Study the drawing (mm; zero at the part's minimum x, y, z) and answer. Round coordinates to 2 decimals unless told otherwise and drop trailing zeros. Write each loop counter-clockwise with the first axis right and the second up, starting at its lowest first coordinate (ties: lowest second). Pieces come first, ordered by that corner, then holes. Notation, with made-up numbers: (87, 0.5) - (96, 0.5) arc R27 ccw to (96, 39.5) - close; hole circle Ø7 at (-16, -8.75). An arc over 180 degrees is marked (long way). Use one line per item in the form item = value. Start each with the question number.
1) The part is cut by section C-C, the plane y = 0.25. Give the vertices of the cut face in (x, z), plus the area to 3 significant figures.
2) This flat-tipped pin is pushed along its axis until it touches: pin 1 (4 mm diameter, centred on x = 30, z = 38.5, fed in from -Y). Where does it stop, or does it pass through?
3) Consider line 1 along Z through (x, y) = (4.5, 0.8); line 2 along Z through (x, y) = (19, 0.95). Determine where each line is inside the solid, lowest interval first. Write a range as from..to.
4) The part is cut by section A-A, the plane x = 4.5. Give the vertices of the cut face in (y, z), plus the area to 3 significant figures.
5) The part is cut by section B-B, the plane z = 3. Give the vertices of the cut face in (x, y).
6) The part is cut by section D-D, the plane x = 15. Give the vertices of the cut face in (y, z), plus the area to 4 significant figures.
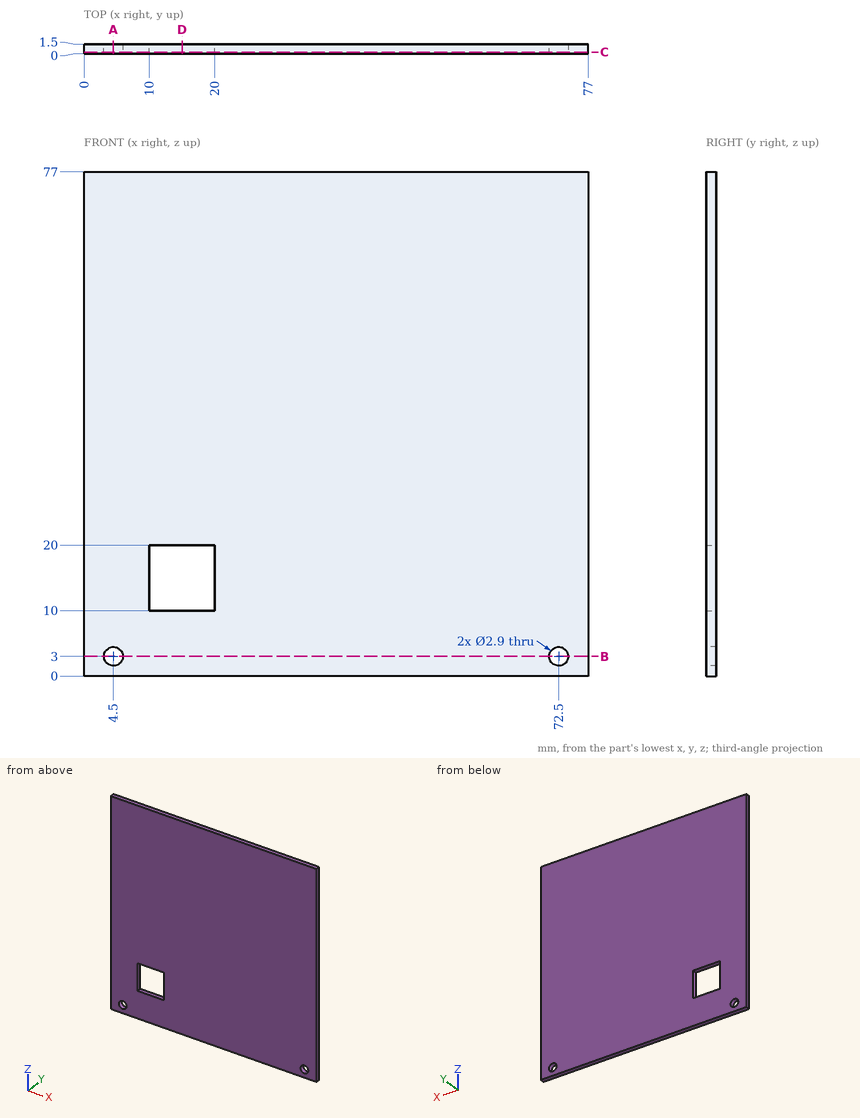
Geometry results:
q1.outline = (0, 0) - (77, 0) - (77, 77) - (0, 77) - close; hole circle Ø2.9 at (4.5, 3); hole (10, 10) - (20, 10) - (20, 20) - (10, 20) - close; hole circle Ø2.9 at (72.5, 3)
q1.area = 5,820 mm2
q2.pin_1 = 0
q3.line_1 = 0..1.55, 4.45..77
q3.line_2 = 0..10, 20..77
q4.outline = (0, 0) - (1.5, 0) - (1.5, 1.55) - (0, 1.55) - close; (0, 4.45) - (1.5, 4.45) - (1.5, 77) - (0, 77) - close
q4.area = 111 mm2
q5.outline = (0, 0) - (3.05, 0) - (3.05, 1.5) - (0, 1.5) - close; (5.95, 0) - (71.05, 0) - (71.05, 1.5) - (5.95, 1.5) - close; (73.95, 0) - (77, 0) - (77, 1.5) - (73.95, 1.5) - close
q6.outline = (0, 0) - (1.5, 0) - (1.5, 10) - (0, 10) - close; (0, 20) - (1.5, 20) - (1.5, 77) - (0, 77) - close
q6.area = 100.5 mm2
